CAD build for the part. Positions are in the model's coordinates, mm. Face numbers are marked on the shaded views. A direction names the side the tool comes from. Give positions to 0.01 mm unless a question says otherwise; leave off trailing zeros. Loops run counter-clockwise (first coordinate to the right, second up) from the corner with the lowest first, then second, coordinate; pieces in that order, holes last.
Item 1: Saw through at A-A on y = -2. Give the cut face in (x, z), plus the area to 3 significant figures.
Item 2: Saw through at B-B on y = -12.25. Give the cut face in (x, z).
Item 3: Which spindle directions (+Z, -Z, +X, -X, +Y, -Y) get a long thin tool onto all of the face, cutting with end or side? Do the marked faces 1 and 2. Say none if no direction does.
Item 4: Probe probe 1 along X at (y, z) = (-2, -65.4); probe 2 along Z at (x, y) = (-20.5, -12.75); probe 3 along Y at (x, z) = (9, -15). List the from-to ranges inside material, lowest first.
Item 5: Drop flat-ended pins along their axis: P1, Ø0.9, axis at y = -6, z = 1.5, coming from the -X side; P2, Ø12, axis at x = 4, z = -7.5, coming from the +Y side; P3, Ø8, axis at x = 1.5, z = -33, coming from the -Y side; P4, Ø4, axis at x = 17.63, y = -9, coming from the -Z side. Give the stop position or say it passes through.
Item 6: Saw through at D-D on z = -29.5. Give the cut face in (x, y), plus the area to 3 significant figures.
Item 7: Saw through at C-C on x = 10. Give the cut face in (y, z).
Autodesk Inventor part; units mm, degrees
ref_plane "YZ Plane" through (0, 0, 0) normal (1, 0, 0) x (0, 1, 0)
ref_plane "XZ Plane" through (0, 0, 0) normal (0, 1, 0) x (-1, 0, 0)
ref_plane "XY Plane" through (0, 0, 0) normal (0, 0, 1) x (1, 0, 0)
sketch "Sketch1" plane through (0, 0, 0) normal (0, 0, 1) x (1, 0, 0)
  line L0 (32.6242, -2.1) -> (40.6242, -2.1)
  arc A0 (41.6242, -3.1) -> (40.6242, -2.1) centre (40.6242, -3.1) ccw
  line L1 (41.6242, -3.1) -> (41.6242, -14)
  line L2 (65.6275, -14) -> (41.6242, -14)
  line L3 (65.6275, -14) -> (65.6275, -2)
  arc A1 (67.6275, 0) -> (65.6275, -2) centre (67.6275, -2) ccw
  line L4 (67.6275, 0) -> (74, 0)
  line L5 (74, 0) -> (74, 2)
  line L6 (10, 2) -> (74, 2)
  line L7 (10, 2) -> (10, -14)
  line L8 (31.6242, -14) -> (10, -14)
  line L9 (31.6242, -14) -> (31.6242, -3.1)
  arc A2 (32.6242, -2.1) -> (31.6242, -3.1) centre (32.6242, -3.1) ccw
  circle A3 centre (12.5, -10.5) radius 1
  circle A4 centre (59.6275, -9) radius 1.5
  circle A5 centre (27.6275, -9) radius 1.5
  circle A6 centre (17.6275, -2) radius 1.5
  circle A7 centre (47.6275, -2) radius 1.5
  circle A8 centre (59.6275, -2) radius 1.5
  circle A9 centre (27.6275, -2) radius 1.5
  circle A10 centre (17.6275, -9) radius 1.5
  circle A11 centre (47.6275, -9) radius 1.5
  line L10 (17.6275, -9) -> (17.6275, -2)
  line L11 (64.6275, -17) -> (10, -17)
  line L12 (20.6275, -13) -> (14.6275, -13)
  line L13 (14.6275, -13) -> (14.6275, 2)
  line L14 (14.6275, 2) -> (20.6275, 2)
  line L15 (20.6275, 2) -> (20.6275, -13)
  line L16 (20.6275, -13) -> (14.6275, 2) construction
  line L17 (14.6275, -13) -> (20.6275, 2) construction
  line L18 (20.6275, -13) -> (14.6275, -13)
  line L19 (14.6275, -13) -> (14.6275, -17)
  line L20 (14.6275, -17) -> (20.6275, -17)
  line L21 (20.6275, -17) -> (20.6275, -13)
  point P0 (0, 0)
  point P1 (17.6275, -5.5)
  dimension "d0" = 6
  dimension "d1" = 15
  dimension "d2" = 6
  dimension "d3" = 4
extrude "Extrusion1" add sketch "Sketch1" along normal blind 3 contours L21 L11 L19 L8 | L8 L19 L12 L21 | L12 L13 L6 L15
ref_plane "Work Plane1" through (-4, 0, -63) normal (0, 0, -1) x (-1, 0, 0)
sketch "Sketch2" plane through (-4, 0, -63) normal (0, 0, -1) x (-1, 0, 0)
  line L0 (32.6242, -2.1) -> (40.6242, -2.1)
  arc A0 (41.6242, -3.1) -> (40.6242, -2.1) centre (40.6242, -3.1) ccw
  line L1 (41.6242, -3.1) -> (41.6242, -14)
  line L2 (65.6275, -14) -> (41.6242, -14)
  line L3 (65.6275, -14) -> (65.6275, -2)
  arc A1 (67.6275, 0) -> (65.6275, -2) centre (67.6275, -2) ccw
  line L4 (67.6275, 0) -> (74, 0)
  line L5 (74, 0) -> (74, 2)
  line L6 (10, 2) -> (74, 2)
  line L7 (10, 2) -> (10, -14)
  line L8 (31.6242, -14) -> (10, -14)
  line L9 (31.6242, -14) -> (31.6242, -3.1)
  arc A2 (32.6242, -2.1) -> (31.6242, -3.1) centre (32.6242, -3.1) ccw
  circle A3 centre (12.5, -10.5) radius 1
  circle A4 centre (59.6275, -9) radius 1.5
  circle A5 centre (27.6275, -9) radius 1.5
  circle A6 centre (17.6275, -2) radius 1.5
  circle A7 centre (47.6275, -2) radius 1.5
  circle A8 centre (59.6275, -2) radius 1.5
  circle A9 centre (27.6275, -2) radius 1.5
  circle A10 centre (17.6275, -9) radius 1.5
  circle A11 centre (47.6275, -9) radius 1.5
  line L10 (64.6275, -17) -> (10, -17)
  line L11 (17.6275, -9) -> (17.6275, -2)
  line L12 (14.6275, -13) -> (20.6275, -13)
  line L13 (20.6275, -13) -> (20.6275, 2)
  line L14 (20.6275, 2) -> (14.6275, 2)
  line L15 (14.6275, 2) -> (14.6275, -13)
  line L16 (14.6275, -13) -> (20.6275, 2) construction
  line L17 (20.6275, -13) -> (14.6275, 2) construction
  line L18 (14.6275, -13) -> (20.6275, -13)
  line L19 (20.6275, -13) -> (20.6275, -17)
  line L20 (20.6275, -17) -> (14.6275, -17)
  line L21 (14.6275, -17) -> (14.6275, -13)
  point P0 (-4, 0)
  point P1 (17.6275, -5.5)
  dimension "d6" = 6
  dimension "d7" = 15
  dimension "d8" = 6
  dimension "d9" = 4
extrude "Extrusion2" add sketch "Sketch2" along normal blind 3 contours L19 L10 L21 L8 | L8 L21 L12 L19 | L12 L15 L6 L13
sketch "Sketch3" plane through (-24.6275, -17, -63) normal (0, -1, 0) x (1, 0, 0)
  line L0 (6, 0) -> (0, 0)
  line L1 (0, 0) -> (0, -3)
  line L2 (6, -3) -> (0, -3)
  line L3 (6, 0) -> (6, -3)
  line L4 (39.255, 63) -> (45.255, 63)
  line L5 (45.255, 63) -> (45.255, 66)
  line L6 (39.255, 66) -> (45.255, 66)
  line L7 (39.255, 63) -> (39.255, 66)
  line L8 (45.255, 63) -> (6, -3)
  line L9 (39.255, 63) -> (39.255, 66)
  line L10 (39.255, 66) -> (0, 0)
  point P0 (24.6275, 63)
extrude "Extrusion3" add sketch "Sketch3" along normal blind 3
fillet "Fillet1" radius 1 2 edges at (14.6275, -17, 1.5) (-18.6275, -17, -64.5)
fillet "Fillet2" radius 2 4 edges at (-18.6275, 2, -64.5) (-24.6275, 2, -64.5) (20.6275, 2, 1.5) (14.6275, 2, 1.5)
properties part number "pcb_holder_3"
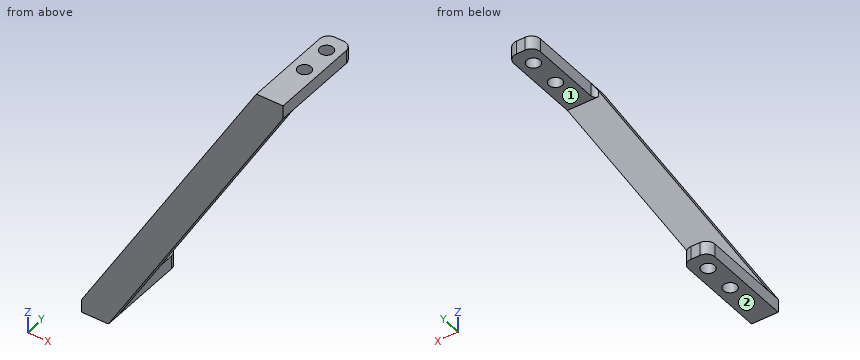
Results below:
1. outline: (-24.63, -66) - (-23.13, -66) - (-23.13, -63) - (-24.63, -63) - close; (-20.13, -66) - (-18.63, -66) - (-18.63, -63) - (-20.13, -63) - close; (14.63, 0) - (16.13, 0) - (16.13, 3) - (14.63, 3) - close; (19.13, 0) - (20.63, 0) - (20.63, 3) - (19.13, 3) - close
1. area: 18.0 mm2
2. outline: (-24.63, -66) - (-18.63, -66) - (-18.63, -63) - (-24.63, -63) - close; (14.63, 0) - (20.63, 0) - (20.63, 3) - (14.63, 3) - close
3. face 1: -Z, +X, -X, +Y
3. face 2: -Z, +X, -X, +Y, -Y
4. probe 1: x = -24.63 to -23.13, -20.13 to -18.63
4. probe 2: z = -66 to -63
4. probe 3: y = -20 to -17
5. P1: stops at x = 14.63
5. P2: stops at y = -17
5. P3: stops at y = -20
5. P4: stops at z = 0
6. outline: (-4.7, -20) - (3.08, -20) - (3.08, -17) - (-4.7, -17) - close
6. area: 23.4 mm2
7. outline: (-20, -17.87) - (-17, -17.87) - (-17, -4.78) - (-20, -4.78) - close
